Work out the finished part from the listing and answer in its coordinate system (mm). Face numbers are marked on the shaded views. A direction names the side the tool comes from. Round coordinates to 2 decimals unless told otherwise and drop trailing zeros. Order: outer loops, then holes, each group sorted by start corner. A loop starts at its lowest first (then second) coordinate and runs counter-clockwise, first axis right, second up. Notation, with made-up numbers: (21, 8) -> (59, 8) arc R23 cw to (59, 39) -> close; hole circle Ø11 at (0, 5.5). An arc over 180 degrees is marked (long way). Use one line per item in the form item = value.
```python
from build123d import *

# Parameters (mm, degrees)
SKETCH2_R           = 1.5
BOSS_EXTRUDE1_DEPTH = 25
FILLET3_R           = 4
FILLET4_R           = 4
FILLET5_R           = 4
FILLET6_R           = 4
FILLET7_R           = 4
FILLET8_R           = 4
FILLET9_R           = 4
FILLET10_R          = 4
CUT_EXTRUDE1_DEPTH  = 10
CUT_EXTRUDE2_DEPTH  = 20
SKETCH5_W           = 19.12768352
SKETCH5_H           = 10.876940682
CUT_EXTRUDE3_DEPTH  = 5
SKETCH6_R           = 10
CUT_EXTRUDE4_DEPTH  = 5


with BuildPart() as part:
    # Sketch2 → Boss-Extrude1 (new body)
    with BuildSketch(Plane(origin=(0, 0, 0), x_dir=(1, 0, 0), z_dir=(0, 1, 0))):
        with BuildLine():
            ThreePointArc((-43.5, 22.5), (-50.328427125, 25.328427125), (-47.5, 18.5))
            Line((-47.5, 18.5), (-47.5, -18.5))
            ThreePointArc((-47.5, -18.5), (-50.328427125, -25.328427125), (-43.5, -22.5))
            Line((-43.5, -22.5), (43.5, -22.5))
            ThreePointArc((43.5, -22.5), (50.328427125, -25.328427125), (47.5, -18.5))
            Line((47.5, -18.5), (47.5, 18.5))
            ThreePointArc((47.5, 18.5), (50.328427125, 25.328427125), (43.5, 22.5))
            Line((43.5, 22.5), (-43.5, 22.5))
        make_face()
        with Locations(Location((-47.5, 22.5, 0), (0, 0, 270))):
            Circle(SKETCH2_R, mode=Mode.SUBTRACT)
        with Locations(Location((-47.5, -22.5, 0), (0, 0, 270))):
            Circle(SKETCH2_R, mode=Mode.SUBTRACT)
        with Locations(Location((47.5, 22.5, 0), (0, 0, 270))):
            Circle(SKETCH2_R, mode=Mode.SUBTRACT)
        with Locations(Location((47.5, -22.5, 0), (0, 0, 270))):
            Circle(SKETCH2_R, mode=Mode.SUBTRACT)
    extrude(amount=BOSS_EXTRUDE1_DEPTH)

    # Fillet3
    fillet3_edges = [part.edges().sort_by_distance(p)[0] for p in [
        (-43.5, 12.5, -22.5),
    ]]
    fillet(fillet3_edges, radius=FILLET3_R)

    # Fillet4
    fillet4_edges = [part.edges().sort_by_distance(p)[0] for p in [
        (-47.5, 12.5, -18.5),
    ]]
    fillet(fillet4_edges, radius=FILLET4_R)

    # Fillet5
    fillet5_edges = [part.edges().sort_by_distance(p)[0] for p in [
        (47.5, 12.5, -18.5),
    ]]
    fillet(fillet5_edges, radius=FILLET5_R)

    # Fillet6
    fillet6_edges = [part.edges().sort_by_distance(p)[0] for p in [
        (43.5, 12.5, -22.5),
    ]]
    fillet(fillet6_edges, radius=FILLET6_R)

    # Fillet7
    fillet7_edges = [part.edges().sort_by_distance(p)[0] for p in [
        (47.5, 12.5, 18.5),
    ]]
    fillet(fillet7_edges, radius=FILLET7_R)

    # Fillet8
    fillet8_edges = [part.edges().sort_by_distance(p)[0] for p in [
        (43.5, 12.5, 22.5),
    ]]
    fillet(fillet8_edges, radius=FILLET8_R)

    # Fillet9
    fillet9_edges = [part.edges().sort_by_distance(p)[0] for p in [
        (-43.5, 12.5, 22.5),
    ]]
    fillet(fillet9_edges, radius=FILLET9_R)

    # Fillet10
    fillet10_edges = [part.edges().sort_by_distance(p)[0] for p in [
        (-47.5, 12.5, 18.5),
    ]]
    fillet(fillet10_edges, radius=FILLET10_R)

    # Sketch3 → Cut-Extrude1 (cut)
    with BuildSketch(Plane(origin=(0, 25, 0), x_dir=(1, 0, 0), z_dir=(0, 1, 0))):
        Polygon((45.159037956, -23.377437582), (47.089402215, -24.96605139), (49.430364258, -24.088613808), (49.840962044, -21.622562418), (47.910597785, -20.03394861), (45.569635742, -20.911386192), align=None)
        Polygon((45.198650859, 21.523377181), (47.1951056, 20.018661771), (49.496454742, 20.99528459), (49.801349141, 23.476622819), (47.8048944, 24.981338229), (45.503545258, 24.00471541), align=None)
        Polygon((-49.801349141, 21.523377181), (-47.8048944, 20.018661771), (-45.503545258, 20.99528459), (-45.198650859, 23.476622819), (-47.1951056, 24.981338229), (-49.496454742, 24.00471541), align=None)
        Polygon((-50, -22.5), (-48.75, -24.665063509), (-46.25, -24.665063509), (-45, -22.5), (-46.25, -20.334936491), (-48.75, -20.334936491), align=None)
    extrude(amount=-CUT_EXTRUDE1_DEPTH, mode=Mode.SUBTRACT)

    # Sketch4 → Cut-Extrude2 (cut)
    with BuildSketch(Plane.XZ):
        with BuildLine():
            Line((-42.5, 15.57179677), (-42.5, -15.57179677))
            ThreePointArc((-42.5, -15.57179677), (-42.568623197, -16.681079599), (-42.77344631, -17.77344631))
            ThreePointArc((-42.77344631, -17.77344631), (-41.681079599, -17.568623197), (-40.57179677, -17.5))
            Line((-40.57179677, -17.5), (40.57179677, -17.5))
            ThreePointArc((40.57179677, -17.5), (41.681079599, -17.568623197), (42.77344631, -17.77344631))
            ThreePointArc((42.77344631, -17.77344631), (42.568623197, -16.681079599), (42.5, -15.57179677))
            Line((42.5, -15.57179677), (42.5, 15.57179677))
            ThreePointArc((42.5, 15.57179677), (42.568623197, 16.681079599), (42.77344631, 17.77344631))
            ThreePointArc((42.77344631, 17.77344631), (41.681079599, 17.568623197), (40.57179677, 17.5))
            Line((40.57179677, 17.5), (-40.57179677, 17.5))
            ThreePointArc((-40.57179677, 17.5), (-41.681079599, 17.568623197), (-42.77344631, 17.77344631))
            ThreePointArc((-42.77344631, 17.77344631), (-42.568623197, 16.681079599), (-42.5, 15.57179677))
        make_face()
    extrude(amount=-CUT_EXTRUDE2_DEPTH, mode=Mode.SUBTRACT)

    # Sketch5 → Cut-Extrude3 (cut)
    with BuildSketch(Plane.ZY.offset(47.5)):
        with Locations((0.337516279, 13.061529659)):
            Rectangle(SKETCH5_W, SKETCH5_H)
    extrude(amount=-CUT_EXTRUDE3_DEPTH, mode=Mode.SUBTRACT)

    # Sketch6 → Cut-Extrude4 (cut)
    with BuildSketch(Plane.XY.offset(22.5)):
        with Locations((26.992807924, 11.532259518)):
            Circle(SKETCH6_R)
    extrude(amount=-CUT_EXTRUDE4_DEPTH, mode=Mode.SUBTRACT)


solid = part.part
```
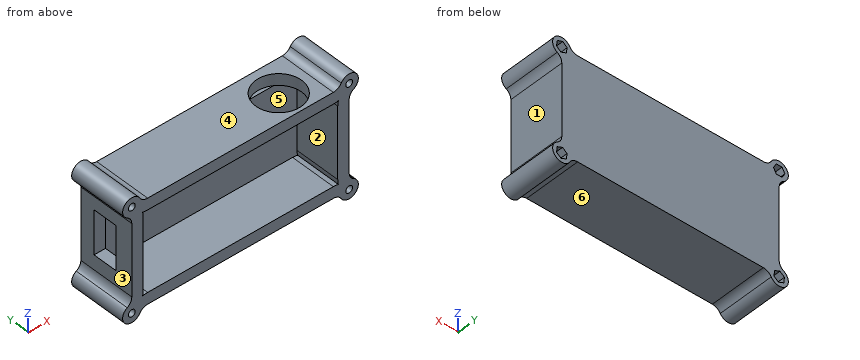
Item 1: Determine the mould class of the marked faces 4, 5 and 6 for opening direction Z: released by +Z, released by -Z, zero draft, split by the parting line, or undercut.
Findings:
face_4 = released by +Z
face_5 = undercut
face_6 = released by -Z
Item 2: The part is cut by section B-B, the plane x = -4.5. Give the vertices of the cut face in (y, z).
Findings:
outline = (0, -22.5) -> (25, -22.5) -> (25, 22.5) -> (0, 22.5) -> (0, 17.5) -> (20, 17.5) -> (20, -17.5) -> (0, -17.5) -> close
Item 3: Flat-ended cylindrical pins translate along their axes: P1, Ø10, axis at x = 15, y = 13, coming from the +Z side; P2, Ø6, axis at y = 5, z = -0.5, coming from the -X side; P3, Ø5, axis at x = -47, z = 21.5, coming from the +Y side; P4, Ø1.4, axis at x = 47.5, z = 22, coming from the +Y side. Find the tip coordinate at first contact, or state that the pin passes through.
Findings:
P1 = 22.5
P2 = -47.5
P3 = 25
P4 = through
Item 4: For the marked faces 1, 2 and 3, determine the directions among +Z, -Z, +X, -X, +Y, -Y from which every point of the face is accessible in a straight line to the end or side of a thin tool.
Findings:
face_1 = +X, +Y, -Y
face_2 = -Y
face_3 = -X, +Y, -Y
Item 5: The part is cut by section A-A, the plane x = 27. Give the vertices of the cut face in (y, z).
Findings:
outline = (0, -22.5) -> (25, -22.5) -> (25, 22.5) -> (21.53, 22.5) -> (21.53, 17.5) -> (20, 17.5) -> (20, -17.5) -> (0, -17.5) -> close; (0, 17.5) -> (1.53, 17.5) -> (1.53, 22.5) -> (0, 22.5) -> close
Item 6: Consider line 1 along Z through (x, y) = (-22.5, 3); line 2 along Y through (x, z) = (14, -12); line 3 along X through (y, z) = (4.75, -13). Determine where each line is inside the solid, lowest interval first.
Findings:
line_1 = -22.5 to -17.5, 17.5 to 22.5
line_2 = 20 to 25
line_3 = -47.5 to -42.5, 42.5 to 47.5
Item 7: The part is cut by section C-C, the plane y = 5.75. Give the number of separate pieces and of enclosed holes in the cut face, and give its area (3 significant figures).
Findings:
separate_pieces = 1
enclosed_holes = 4
area = 1,350 mm^2
